from build123d import *


with BuildPart() as part:
    # Sketch → Revolution (revolve)
    with BuildSketch(Plane.XZ):
        with BuildLine():
            Line((2.7, 0), (2.7, 22))
            Line((2.7, 22), (0, 27))
            Line((0, 27), (0, 118))
            Line((0, 118), (1.570833, 114.42474))
            ThreePointArc((2.5, 110), (2.265202, 112.260624), (1.570833, 114.42474))
            Line((2.5, 110), (2.5, 29.65414))
            ThreePointArc((2.5, 29.65414), (2.62833, 28.531812), (3.006695, 27.46742))
            Line((3.006695, 27.46742), (3.832075, 25.78202))
            ThreePointArc((4.7, 22.036358), (4.480182, 23.958809), (3.832075, 25.78202))
            Line((4.7, 22.036358), (4.7, 0))
            Line((4.7, 0), (2.7, 0))
        make_face()
    revolve(axis=Axis((0, 0, 0), (0, 0, 1)))


solid = part.part
Verification items for the finished model (mm, model axes). A direction names the side the tool comes from. Coordinates: 2 decimals unless noted, no trailing zeros. Loops run counter-clockwise (first coordinate to the right, second up) from the corner with the lowest first, then second, coordinate; pieces in that order, holes last. Notation, with made-up numbers: (61, 85) -> (84, 85) arc R17 ccw to (84, 99) -> close; hole circle Ø4 at (69.25, 65.5). An arc over 180 degrees is marked (long way). Answer as a JSON object with one key per item and string values. Group by question number.
Item 1: Sectioned sample at B-B on z = 59. Record the boundary of the cut face in (x, y).
Item 2: Scan lines: probe 1 along Y at (x, z) = (0, 15.25); probe 2 along Y at (x, z) = (1.5, 20.5) (3 decimals); probe 3 along Z at (x, y) = (-2.75, 2.5). Record each from-to range of solid material in increasing order.
Item 3: Mould release check, pull along Y, two halves, no side actions. Record for faces 1 (the flat face through (2.02, -2.02, 0)), 2 (the cylindrical face through (-1.02, -4.59, 10.86)), 3 (the conical face through (-0.818, -0.627, 25.091)): +Y half, -Y half, draft (parallel to the pull), parting line (faces both ways), or undercut.
Item 4: Sectioned sample at A-A on z = 11. Record the boundary of the cut face in (x, y), plus the area to 3 significant figures.
Item 5: Tool access check on faces 4 (the cylindrical face through (-0.585, -2.636, 11.154)), 5 (the cylindrical face through (-0.54, -2.44, 69.26)). Record the directions out of +Z, -Z, +X, -X, +Y, -Y that give a thin tool (end or side, any length) a straight path to the whole face; none if there is none.
Evaluation:
{
 "1": {"outline": "circle Ø5 at (0, 0)"},
 "2": {"probe 1": "y = -4.7 to -2.7, 2.7 to 4.7", "probe 2": "y = -4.454 to -2.245, 2.245 to 4.454", "probe 3": "z = 0 to 26.02"},
 "3": {"face 1": "draft", "face 2": "parting line", "face 3": "undercut"},
 "4": {"outline": "circle Ø9.4 at (0, 0); hole circle Ø5.4 at (0, 0)", "area": "46.5 mm²"},
 "5": {"face 4": "-Z", "face 5": "+Z"}
}
